Verification items for this drawing (mm, ordinates from the low corner). A direction names the side the tool comes from. Round coordinates to 2 decimals unless told otherwise and drop trailing zeros. Loops run counter-clockwise (first coordinate to the right, second up) from the corner with the lowest first, then second, coordinate; pieces in that order, holes last. Notation, with made-up numbers: M 14,37 L 18,37 A20 cw 18,59 Z; hole C 33,76.25 d3. An arc over 180 degrees is marked long. One line per item, written item: value.
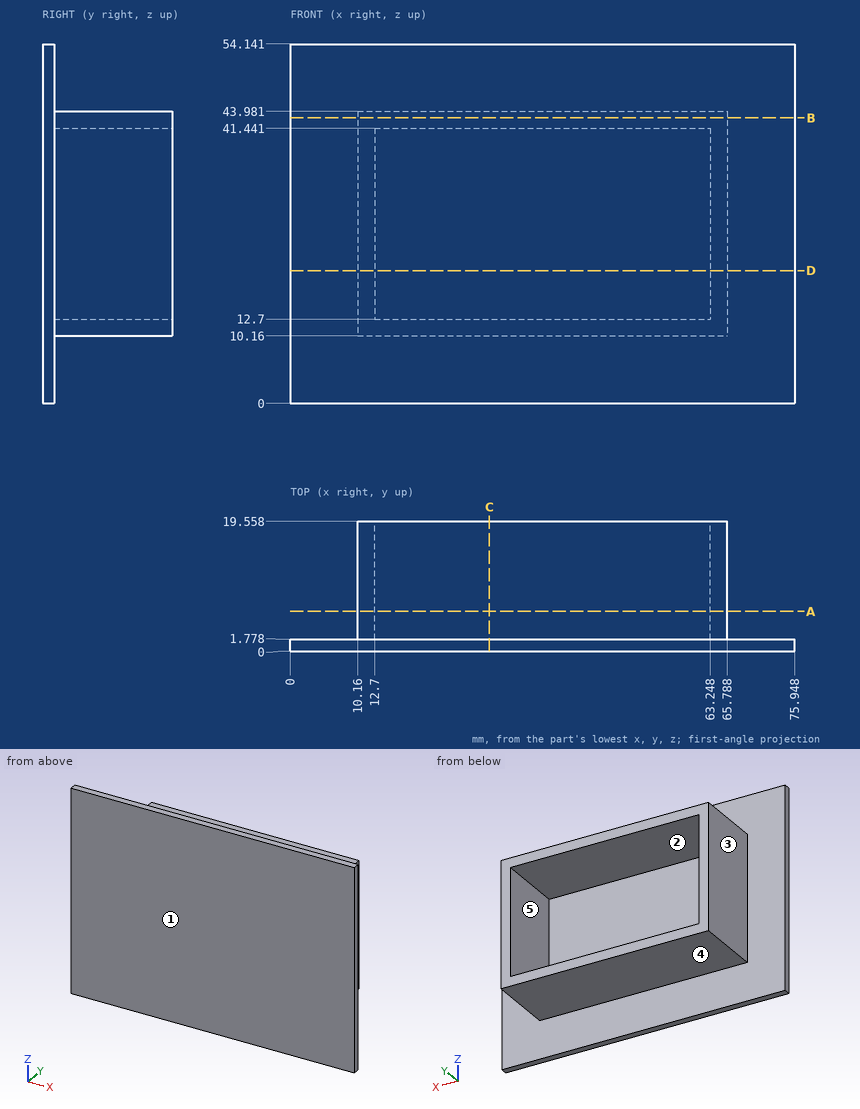
(1) Sectioned sample at D-D on z = 20. Enter the section's corners in (x, y).
Completed:
outline: M 0,0 L 75.95,0 L 75.95,1.78 L 65.79,1.78 L 65.79,19.56 L 63.25,19.56 L 63.25,1.78 L 12.7,1.78 L 12.7,19.56 L 10.16,19.56 L 10.16,1.78 L 0,1.78 Z
(2) Thickness scan on L1, parallel to X at y = 13, z = 15; L2, parallel to Z at x = 27, y = 14.75; L3, parallel to Y at x = 49, z = 7. Record the ranges inside material, lowest first. Write a range as from..to.
Completed:
L1: x = 10.16..12.7, 63.25..65.79
L2: z = 10.16..12.7, 41.44..43.98
L3: y = 0..1.78
(3) Sectioned sample at B-B on z = 43. Enter the section's corners in (x, y), and give its area (3 significant figures).
Completed:
outline: M 0,0 L 75.95,0 L 75.95,1.78 L 65.79,1.78 L 65.79,19.56 L 10.16,19.56 L 10.16,1.78 L 0,1.78 Z
area: 1,120 mm^2
(4) Sectioned sample at C-C on x = 30. Enter the section's corners in (y, z).
Completed:
outline: M 0,0 L 1.78,0 L 1.78,10.16 L 19.56,10.16 L 19.56,12.7 L 1.78,12.7 L 1.78,41.44 L 19.56,41.44 L 19.56,43.98 L 1.78,43.98 L 1.78,54.14 L 0,54.14 Z
(5) Mould release check, pull along X, two halves, no side actions. Record for the marked faces 3, 4 and 5: +X half, -X half, draft (parallel to the pull), parting line (faces both ways), or undercut.
Completed:
face 3: -X half
face 4: draft
face 5: undercut
(6) Tool access check on the marked faces 1 and 2. Record the directions out of +Z, -Z, +X, -X, +Y, -Y that give a thin tool (end or side, any length) a straight path to the whole face; none if there is none.
Completed:
face 1: +Z, -Z, +X, -X, -Y
face 2: +Y
(7) Depth check by flat-ended pin: pin 1 Ø1.5 at (y, z) = (10, 23.5) entering from +X; pin 2 Ø10 at (x, z) = (66.5, 36) entering from +Y; pin 3 Ø3 at (y, z) = (6.5, 33.5) entering from -X; pin 4 Ø5 at (x, y) = (35, 11.5) entering from -Z. Enter the tip coordinate at first touch or a pass-through.
Completed:
pin 1: stops at x = 65.79
pin 2: stops at y = 19.56
pin 3: stops at x = 10.16
pin 4: stops at z = 10.16
(8) Sectioned sample at A-A on y = 6. Enter the section's corners in (x, z).
Completed:
outline: M 10.16,10.16 L 65.79,10.16 L 65.79,43.98 L 10.16,43.98 Z; hole M 12.7,12.7 L 63.25,12.7 L 63.25,41.44 L 12.7,41.44 Z
